Could you check a few things on this model? Use its own coordinates, in mm. Round coordinates to 2 decimals unless told otherwise and drop trailing zeros. Order: outer loops, then holes, each group sorted by start corner. A loop starts at its lowest first (then second) coordinate and runs counter-clockwise, first axis right, second up. Notation, with made-up numbers: (7, 83.25) - (53, 83.25) arc R7 cw to (53, 96.25) - close; hole circle Ø9 at (56.25, -14). An arc over 180 degrees is marked (long way). Use one line per item in the form item = value.
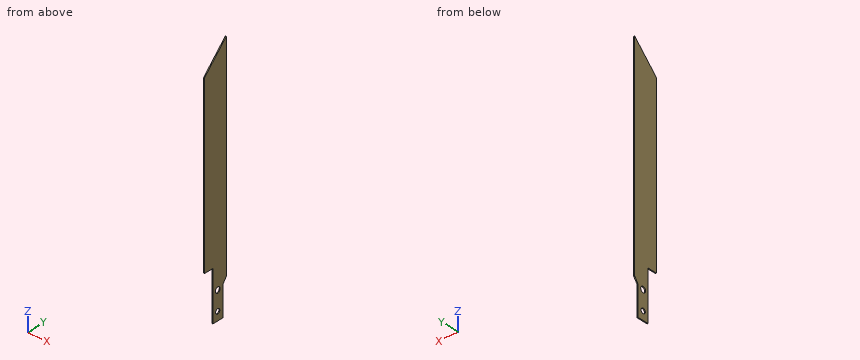
from build123d import *

# Parameters (mm, degrees)
F0_R     = 4.973557
F0_R_2   = 5.819766
F1_DEPTH = 1.89738
F2_DEPTH = 1.89738
F5_DEPTH = 25.4
F6_W     = 20.362974
F6_H     = 103.774652
F7_DEPTH = 1.89838


with BuildPart() as f1:
    # F0 (on Right) → F1 (new body)
    with BuildSketch(Plane.YZ):
        Polygon((20.065772, -302.329028), (20.065772, 205.670972), (-30.734228, 154.870972), (-30.734228, -302.329028), align=None)
        with Locations((0, -284.892797)):
            Circle(F0_R, mode=Mode.SUBTRACT)
        with Locations((0, -246.153131)):
            Circle(F0_R_2, mode=Mode.SUBTRACT)
    extrude(amount=F1_DEPTH)

    # F0 (on Right) → F2 (join)
    with BuildSketch(Plane.YZ):
        Polygon((20.065772, -302.329028), (20.065772, 205.670972), (-30.734228, 154.870972), (-30.734228, -302.329028), align=None)
        with Locations((0, -284.892797)):
            Circle(F0_R, mode=Mode.SUBTRACT)
        with Locations((0, -246.153131)):
            Circle(F0_R_2, mode=Mode.SUBTRACT)
    extrude(amount=F2_DEPTH)

    # F4 (on face) → F5 (cut)
    with BuildSketch(Plane.YZ.offset(1.89738)):
        Polygon((-30.734228, -234.08674), (-31.288195, -233.662769), (-31.288195, -303.030223), (-19.98027, -303.18138), (-19.98027, -302.329028), (-30.734228, -302.329028), align=None)
        Polygon((20.065772, -302.329028), (11.948531, -302.329028), (11.948531, -303.18138), (20.324497, -303.18138), (20.928504, -229.346052), (20.065772, -230.59222), align=None)
        Polygon((11.948531, -242.317125), (11.948531, -302.329028), (20.065772, -302.329028), (20.065772, -230.59222), align=None)
        Polygon((-19.98027, -242.317125), (-30.734228, -234.08674), (-30.734228, -302.329028), (-19.98027, -302.329028), align=None)
    extrude(amount=-F5_DEPTH, mode=Mode.SUBTRACT)

    # F6 (on Right) → F7 (cut, through all)
    with BuildSketch(Plane.YZ):
        with Locations((-21.773375, -253.215976)):
            Rectangle(F6_W, F6_H)
    extrude(amount=F7_DEPTH, mode=Mode.SUBTRACT)


solid = f1.part
Item 1: Will these pins go through, and if not, where does the flat tip stop? P1, Ø0.6, axis at x = 0.5, y = -20.5, coming from the -Z side; P2, Ø7, axis at y = 0, z = -246.15, coming from the -X side (1 decimal).
Found:
P1 = -201.33
P2 = through
Item 2: I need wall thicknesses on L1, parallel to Z at x = 1, y = -3.5; L2, parallel to Y at x = 1.5, z = -205; L3, parallel to Z at x = 1.4, y = 0. Which ranges of each line are inside material? Lowest first, please.
Found:
L1 = -302.33 to -288.43, -281.36 to -250.8, -241.5 to 182.11
L2 = -11.59 to 20.07
L3 = -302.33 to -289.87, -279.92 to -251.97, -240.33 to 185.61
Item 3: Imagine slicing it at C-C on z = -223.5. Please give me the cut outline in (x, y).
Found:
outline = (0, -11.59) - (1.9, -11.59) - (1.9, 20.07) - (0, 20.07) - close
Item 4: Imagine slicing it at A-A on y = 0. Please give me the cut outline in (x, z).
Found:
outline = (0, -302.33) - (1.9, -302.33) - (1.9, -289.87) - (0, -289.87) - close; (0, -279.92) - (1.9, -279.92) - (1.9, -251.97) - (0, -251.97) - close; (0, -240.33) - (1.9, -240.33) - (1.9, 185.61) - (0, 185.61) - close
Item 5: Imagine slicing it at B-B on x = 1.2. Please give me the cut outline in (y, z).
Found:
outline = (-30.73, -201.33) - (-11.59, -201.33) - (-11.59, -302.33) - (11.95, -302.33) - (11.95, -242.32) - (20.07, -230.59) - (20.07, 205.67) - (-30.73, 154.87) - close; hole circle Ø11.64 at (0, -246.15); hole circle Ø9.95 at (0, -284.89)
